Verification items for the finished model (mm, model axes). A direction names the side the tool comes from. Coordinates: 2 decimals unless noted, no trailing zeros. Loops run counter-clockwise (first coordinate to the right, second up) from the corner with the lowest first, then second, coordinate; pieces in that order, holes last. Notation, with made-up numbers: (-27, -21.5) -> (-6, -21.5) arc R23 ccw to (-6, 10.5) -> close; hole circle Ø3 at (19, 12.25). An arc over 180 degrees is marked (long way). Answer as a JSON object with one key per item and string values. Group by question number.
Q1. Cross-section at A-A on x = -19.05. Record the boundary of the cut face in (y, z) (3 decimals).
Q2. Release check for a two-part mould opening along Z. For faces 1 (the flat face through (-16, -19.05, -1)), 2 (the flat face through (-2, -10, -82.55)), 3 (the cylindrical face through (-12.485, -17.485, -14.337)) record: released by +Z, released by -Z, zero draft, split by the parting line, or undercut.
Q3. Cross-section at C-C on z = 46.5. Record the boundary of the cut face in (x, y) (3 decimals), and give its area (3 significant figures).
Q4. Scan lines: L1, parallel to Z at x = -12.7, y = -16.8; L2, parallel to Z at x = -19.05, y = -16.9; L3, parallel to Y at x = -13.25, z = -49 (3 decimals). Record each from-to range of solid material in increasing order.
Q5. Cross-section at B-B on z = 76.2. Record the boundary of the cut face in (x, y) (3 decimals).
Q6. Cross-section at D-D on y = 0. Record the boundary of the cut face in (x, z) (3 decimals).
Q7. Set-up check for faces 4 (the flat face through (-2, -10, 82.55)), 5 (the flat face through (-3.175, 0, 1)): record each of +Z, -Z, +X, -X, +Y, -Y from which the full face is reachable in a straight line by a thin tool's end or side.
Q8. Gauge pin test, flat ends, axial feed: pin 1 Ø5.5 at (x, z) = (-19.05, -50.8) entering from +Y (3 decimals); pin 2 Ø7.5 at (y, z) = (-6, 12) entering from -X (3 decimals); pin 3 Ø3 at (x, z) = (-6.5, 51) entering from +Y. Record the tip position at first contact, or that the pin passes through.
```python
from build123d import *

# Parameters (mm, degrees)
SKETCH2_W                   = 165.1
SKETCH2_H                   = 25.4
BASE_FLANGE1_DEPTH          = 3.175
EDGE_FLANGE1_DEPTH          = 165.1
F_1_8_0_13_DIAMETER_HOLE1_D = 3.302


# Sheet-metal steps are written as plain solids
with BuildPart() as part:
    # Sketch2 → Base-Flange1 (new body)
    with BuildSketch(Plane(origin=(0, 0, 0), x_dir=(0, 0, -1), z_dir=(1, 0, 0))):
        Rectangle(SKETCH2_W, SKETCH2_H)
    extrude(amount=-BASE_FLANGE1_DEPTH)

    # Edge-Flange1 section (across the edge) → Edge-Flange1 (add)
    with BuildSketch(Plane(origin=(-3.175, -15.875, -82.55), x_dir=(0, 1, 0), z_dir=(0, 0, 1))):
        with BuildLine():
            Line((-3.175, 3.175), (-3.175, 22.225))
            Line((-3.175, 22.225), (0, 22.225))
            Line((0, 22.225), (0, 3.175))
            ThreePointArc((0, 3.175), (0.92993597, 0.92993597), (3.175, 0))
            Line((3.175, 0), (3.175, -3.175))
            ThreePointArc((3.175, -3.175), (-1.315128061, -1.315128061), (-3.175, 3.175))
        make_face()
    extrude(amount=EDGE_FLANGE1_DEPTH)

    # 1/8 (0.13) Diameter Hole1 (through all)
    with Locations(Plane(origin=(0, -15.875, 0), x_dir=(1, 0, 0), z_dir=(0, 1, 0))):
        with Locations((-12.7, 76.2), (-19.05, 50.8), (-12.7, 12.7), (-19.05, -12.7), (-12.7, -50.8), (-19.05, -76.2)):
            Hole(F_1_8_0_13_DIAMETER_HOLE1_D / 2)


solid = part.part
```
Computed values:
{
 "1": {"outline": "(-19.05, -82.55) -> (-15.875, -82.55) -> (-15.875, -52.451) -> (-19.05, -52.451) -> close; (-19.05, -49.149) -> (-15.875, -49.149) -> (-15.875, 11.049) -> (-19.05, 11.049) -> close; (-19.05, 14.351) -> (-15.875, 14.351) -> (-15.875, 74.549) -> (-19.05, 74.549) -> close; (-19.05, 77.851) -> (-15.875, 77.851) -> (-15.875, 82.55) -> (-19.05, 82.55) -> close"},
 "2": {"face 1": "zero draft", "face 2": "released by -Z", "face 3": "undercut"},
 "3": {"outline": "(-25.4, -19.05) -> (-6.35, -19.05) arc R6.35 ccw to (0, -12.7) -> (0, 12.7) -> (-3.175, 12.7) -> (-3.175, -12.7) arc R3.175 cw to (-6.35, -15.875) -> (-25.4, -15.875) -> close", "area": "165 mm²"},
 "4": {"L1": "z = -82.55 to -77.85, -74.55 to -14.35, -11.05 to 49.15, 52.45 to 82.55", "L2": "z = -82.55 to -52.45, -49.15 to 11.05, 14.35 to 74.55, 77.85 to 82.55", "L3": "y = -19.05 to -15.875"},
 "5": {"outline": "(-25.4, -19.05) -> (-20.701, -19.05) -> (-20.701, -15.875) -> (-25.4, -15.875) -> close; (-17.399, -19.05) -> (-6.35, -19.05) arc R6.35 ccw to (0, -12.7) -> (0, 12.7) -> (-3.175, 12.7) -> (-3.175, -12.7) arc R3.175 cw to (-6.35, -15.875) -> (-17.399, -15.875) -> close"},
 "6": {"outline": "(-3.175, -82.55) -> (0, -82.55) -> (0, 82.55) -> (-3.175, 82.55) -> close"},
 "7": {"face 4": "+Z, +X, -X, +Y, -Y", "face 5": "+Z, -Z, -X, +Y"},
 "8": {"pin 1": "stops at y = -15.875", "pin 2": "stops at x = -3.175", "pin 3": "stops at y = -15.57"}
}
